Source: CAD feature listing. Evaluate the final solid. Frame: model axes, mm. A direction names the side the tool comes from. Round coordinates to 2 decimals unless told otherwise and drop trailing zeros. Write each loop counter-clockwise with the first axis right and the second up, starting at its lowest first coordinate (ties: lowest second). Pieces come first, ordered by that corner, then holes. Notation, with made-up numbers: M 16.5,-15 L 45.5,-15 A14 ccw 45.5,4 Z; hole C 43.5,21.5 d8. An arc over 180 degrees is marked long. Answer in a Markdown table with one row per item. Add a question column.
Item 1: Cut plane A-A on z = 694. Return loops of the section in (x, y).
Item 2: Mould query, pull axis Y, two halves, no side actions, for faces 1 (the face through (138, 141.354, 499)), 2 (the face through (0, 6, 579)), 3 (the face through (99.32, 292.61, 123.25)). Classes: released by +Y, released by -Y, zero draft, split by the parting line, or undercut.
Item 3: Contact query for flat-ended pins moving along their axis: pin 1 (5 mm diameter, centred on x = 224.5, y = 148.5, fed in from +Z); pin 2 (2 mm diameter, centred on x = 96, y = 409.5, fed in from -Z); pin 3 (15.5 mm diameter, centred on x = 21.5, z = 378.5, fed in from +Y). Output: stop coordinate, or through.
Item 4: Material intervals for probe 1 along X at (y, z) = (-30.5, 420); probe 2 along Y at (x, z) = (139, 439); probe 3 along Y at (x, z) = (174.5, 663.5), sorted ascending.
Item 5: Cut plane B-B on y = -34.5. Return loops of the section in (x, z).
Item 6: Cut plane C-C on z = 200. Return loops of the section in (x, y).
Item 7: Set-up query: faces 4 (the face through (268, 129.114, 393)), 5 (the face through (220.301, 143, 123)), 6 (the face through (308.326, 112.02, 785.507)). Return all of +Z, -Z, +X, -X, +Y, -Y with unobstructed straight access to the full face (end or side cutting, diameter ignored); none if empty.
Item 8: Cut plane D-D on y = 479. Return loops of the section in (x, z), and give its area (3 significant figures).
from build123d import *

# Parameters (mm, degrees)
PAD_DEPTH       = 300
POCKET_DEPTH    = 488.796135
SKETCH002_W     = 818.782761
SKETCH002_H     = 489.886894
POCKET001_DEPTH = 250
POCKET002_DEPTH = 732.016625
PAD001_DEPTH    = 20
PAD002_DEPTH    = 60
SKETCH006_R     = 24.969388
PAD003_DEPTH    = 10


with BuildPart() as part:
    # Sketch → Pad (new body)
    with BuildSketch(Plane.YZ):
        Polygon((0, 0), (-19.795493, 299.346185), (-123.951116, 355.086699), (-123.951116, 815.086699), (101.470154, 815.086699), (101.470154, 464.449951), (133.118958, 464.449951), (142.856949, 488.795135), (598.112183, 488.795135), (593.243164, 334.823194), (513.112758, 334.823194), (317.295496, 246.798924), (302.479552, 0), align=None)
    extrude(amount=PAD_DEPTH)

    # Sketch001 (on Face3 of Pad) → Pocket (cut, through all)
    with BuildSketch(Plane(origin=(0, 0, 488.795135), x_dir=(0, -1, 0), z_dir=(0, 0, 1))):
        with BuildLine():
            Line((-398.685885, 289.727159), (-579.183769, 208.886406))
            ThreePointArc((-579.183769, 208.886406), (-593.86479, 196.305532), (-599.345764, 177.764505))
            Line((-599.345764, 177.764505), (-599.345764, 114.282631))
            ThreePointArc((-599.345764, 114.282631), (-596.613394, 105.037965), (-589.294345, 98.764115))
            Line((-589.294345, 98.764115), (-390.579573, 9.719232))
            ThreePointArc((-390.579573, 9.719232), (-368.364571, 2.45696), (-345.122148, 0))
            Line((-345.122148, 0), (-228.797617, 0))
            ThreePointArc((-228.797617, 0), (-216.966667, 1.836648), (-206.24937, 7.173706))
            Line((-206.24937, 7.173706), (-143.517624, 51.585079))
            Line((-143.517624, 51.585079), (-131.65593, 52.432343))
            Line((-131.65593, 52.432343), (-131.65593, -48.39209))
            Line((-131.65593, -48.39209), (-645.098022, -48.39209))
            Line((-645.098022, -48.39209), (-645.098022, 347.280304))
            Line((-645.098022, 347.280304), (-129.11412, 347.280304))
            Line((-129.11412, 347.280304), (-129.11412, 246.455841))
            Line((-129.11412, 246.455841), (-142.67038, 245.608597))
            Line((-142.67038, 245.608597), (-196.823145, 282.503901))
            ThreePointArc((-196.823145, 282.503901), (-221.003748, 294.141504), (-247.539678, 298.138977))
            Line((-247.539678, 298.138977), (-359.325075, 298.138977))
            ThreePointArc((-359.325075, 298.138977), (-379.449886, 296.012544), (-398.685885, 289.727159))
        make_face()
    extrude(amount=-POCKET_DEPTH, mode=Mode.SUBTRACT)

    # Sketch002 (on Face10 of Pocket) → Pocket001 (cut)
    with BuildSketch(Plane.YX):
        with Locations((231.305886, 120.791111)):
            Rectangle(SKETCH002_W, SKETCH002_H)
        with BuildLine():
            Line((-19.853376, 184.187614), (-19.853376, 108.753578))
            ThreePointArc((-19.853376, 108.753578), (-12.888522, 91.938931), (3.926125, 84.974077))
            Line((3.926125, 84.974077), (257.438717, 84.974077))
            ThreePointArc((257.438717, 84.974077), (292.99976, 99.703943), (307.729626, 135.264986))
            Line((307.729626, 135.264986), (307.729626, 178.492494))
            ThreePointArc((307.729626, 178.492494), (295.484184, 208.055606), (265.921072, 220.301047))
            Line((265.921072, 220.301047), (16.260057, 220.301047))
            ThreePointArc((16.260057, 220.301047), (-9.275997, 209.723668), (-19.853376, 184.187614))
        make_face(mode=Mode.SUBTRACT)
    extrude(amount=-POCKET001_DEPTH, mode=Mode.SUBTRACT)

    # Sketch003 (on Face37 of Pocket001) → Pocket002 (cut, through all)
    with BuildSketch(Plane(origin=(0, 582.073055, -18.406761), x_dir=(0, 0.031607, 0.9995), z_dir=(0, 0.9995, -0.031607))):
        Polygon((435.498799, 463.280181), (-86.974939, 463.280181), (-86.974939, 225.514861), (240.394508, 225.514861), (435.498799, 323.83508), align=None)
        Polygon((-86.974939, -130.245743), (441.643773, -130.245743), (441.643773, -18.749703), (232.713184, 81.106918), (-86.974939, 81.106918), align=None)
    extrude(amount=-POCKET002_DEPTH, mode=Mode.SUBTRACT)

    # Sketch004 (on Face13 of Pocket002) → Pad001 (join)
    with BuildSketch(Plane(origin=(0, 0, 488.795135), x_dir=(0, -1, 0), z_dir=(0, 0, 1))):
        with BuildLine():
            Line((-171.192747, 274.879835), (-205.725164, 301.3696))
            ThreePointArc((-205.725164, 301.3696), (-218.875285, 308.396663), (-233.586133, 310.82489))
            Line((-233.586133, 310.82489), (-379.426666, 310.82489))
            ThreePointArc((-379.426666, 310.82489), (-394.200864, 309.220658), (-408.286409, 304.482739))
            Line((-408.286409, 304.482739), (-596.739704, 217.45158))
            ThreePointArc((-596.739704, 217.45158), (-610.910495, 205.093416), (-616.18866, 187.046905))
            Line((-616.18866, 187.046905), (-616.18866, 112.117576))
            ThreePointArc((-616.18866, 112.117576), (-610.808276, 94.401768), (-596.484569, 82.670196))
            Line((-596.484569, 82.670196), (-395.775735, -0.157481))
            ThreePointArc((-395.775735, -0.157481), (-370.410961, -7.824527), (-344.039491, -10.413148))
            Line((-344.039491, -10.413148), (-224.040587, -10.413148))
            ThreePointArc((-224.040587, -10.413148), (-208.179544, -7.736142), (-194.07573, -0.001706))
            Line((-194.07573, -0.001706), (-159.302641, 27.480226))
            ThreePointArc((-159.302641, 27.480226), (-146.077517, 43.952537), (-141.354309, 64.542152))
            Line((-141.354309, 64.542152), (-141.354309, 214.384436))
            ThreePointArc((-141.354309, 214.384436), (-149.219607, 248.111375), (-171.192747, 274.879835))
        make_face()
    extrude(amount=PAD001_DEPTH)

    # Sketch005 (on Face12 of Pad001) → Pad002 (join)
    with BuildSketch(Plane(origin=(0, 0, 815.086699), x_dir=(0, -1, 0), z_dir=(0, 0, 1))):
        with BuildLine():
            Line((-121.608505, 285.532054), (-121.608505, 32.202011))
            ThreePointArc((-121.608505, 32.202011), (-106.07924, -5.28895), (-68.58828, -20.818214))
            Line((-68.58828, -20.818214), (87.40585, -20.818214))
            ThreePointArc((87.40585, -20.818214), (127.524005, -4.20073), (144.141488, 35.917424))
            Line((144.141488, 35.917424), (144.141488, 270.594498))
            ThreePointArc((144.141488, 270.594498), (130.426894, 303.704458), (97.316935, 317.419052))
            Line((97.316935, 317.419052), (-89.721507, 317.419052))
            ThreePointArc((-89.721507, 317.419052), (-112.269019, 308.079566), (-121.608505, 285.532054))
        make_face()
    extrude(amount=-PAD002_DEPTH)

    # Sketch006 (on Face70 of Pad002) → Pad003 (join)
    with BuildSketch(Plane(origin=(0, 0, 815.086699), x_dir=(0, -1, 0), z_dir=(0, 0, 1))):
        with Locations((24.969388, 148.605312)):
            Circle(SKETCH006_R)
    extrude(amount=PAD003_DEPTH)


solid = part.part
Results below:
| question | item | result |
|---|---|---|
| 1 | outline | M 0,-123.95 L 300,-123.95 L 300,101.47 L 0,101.47 Z |
| 2 | face 1 | undercut |
| 2 | face 2 | zero draft |
| 2 | face 3 | released by +Y |
| 3 | pin 1 | z = 508.8 |
| 3 | pin 2 | z = 287.8 |
| 3 | pin 3 | y = 434.16 |
| 4 | probe 1 | 0 to 300 |
| 4 | probe 2 | -123.95 to 596.54 |
| 4 | probe 3 | -123.95 to 101.47 |
| 5 | outline | M -20.82,755.09 L 0,755.09 L 0,403.71 L 46.09,307.22 L 258.56,307.22 L 300,389.49 L 300,755.09 L 317.42,755.09 L 317.42,815.09 L 171.68,815.09 L 171.68,825.09 L 125.53,825.09 L 125.53,815.09 L -20.82,815.09 Z |
| 6 | outline | M 84.97,3.93 A23.78 ccw 92.28,-13.23 L 205.04,-13.23 A36.11 ccw 220.3,16.26 L 220.3,265.92 A41.81 ccw 178.49,307.73 L 135.26,307.73 A50.29 ccw 84.97,257.44 Z |
| 7 | face 4 | +Z, -Z, +X |
| 7 | face 5 | -Z, +X, +Y, -Y |
| 7 | face 6 | +Z, +X, +Y |
| 8 | outline | M 34.19,488.8 L 49.34,488.8 L 49.34,319.49 L 253.76,319.49 L 253.76,488.8 L 271.83,488.8 L 271.83,508.8 L 34.19,508.8 Z |
| 8 | area | 39,400 mm2 |
